Autodesk Inventor part; units mm, degrees
ref_plane "Plano de trabalho1" through (-163.24, 6, 12.15) normal (0, 0, 1) x (1, 0, 0)
ref_plane "Plano de trabalho2" through (-39.87, 6, 5) normal (0, 0, 1) x (1, 0, 0)
ref_plane "YZ Plane" through (0, 0, 0) normal (1, 0, 0) x (0, 1, 0)
sketch "Esboço1" plane through (0, 0, 0) normal (0, 1, 0) x (-1, 0, 0)
  line L0 (0, 5) -> (39.87, 5)
  line L1 (39.87, 5) -> (39.87, 12.15)
  line L2 (39.87, 12.15) -> (163.24, 12.15)
  line L3 (163.24, 12.15) -> (163.24, 7.27)
  line L4 (163.24, 7.27) -> (43.67, 7.27)
  line L5 (43.67, 7.27) -> (43.67, -0.21)
  line L6 (43.67, -0.21) -> (0, -0.21)
  line L7 (0, 5) -> (2.5, 5) construction
  line L8 (2.5, 5) -> (2.5, 1.56) construction
  line L9 (2.5, 1.56) -> (0, 1.56) construction
  line L10 (2.5, 1.56) -> (0, 5)
  line L11 (2.5, 1.56) -> (0, 1.56)
  line L12 (0, 1.56) -> (0, -0.21)
  point P0 (0, 0)
  dimension "d0" = 39.87
  dimension "d1" = 7.15
  dimension "d2" = 123.37
  dimension "d3" = 4.88
  dimension "d4" = 119.57
  dimension "d5" = 7.48
  dimension "d6" = 2.5
  dimension "d7" = 3.44
  dimension "d8" = 5.21
extrude "Extrusão1" add sketch "Esboço1" along normal mid plane 12
ref_plane "Plano de trabalho1" through (-163.24, 6, 12.15) normal (0, 0, 1) x (1, 0, 0)
ref_plane "Plano de trabalho2" through (-39.87, 6, 5) normal (0, 0, 1) x (1, 0, 0)
sketch "Esboço2" plane through (-163.24, 6, 12.15) normal (0, 0, 1) x (1, 0, 0)
  line L0 (123.37, 0) -> (123.37, -12) construction
  line L1 (123.37, -6) -> (110.26, -6) construction
  line L2 (0, 0) -> (0, -12) construction
  line L3 (0, -6) -> (3.56, -6) construction
  line L4 (110.26, -6) -> (0, -6) construction
  line L5 (3.56, -6) -> (110.26, -6) construction
  line L6 (6.785, -9.225) -> (107.035, -9.225)
  line L7 (107.035, -2.775) -> (6.785, -2.775)
  arc A0 (6.785, -2.775) -> (6.785, -9.225) centre (6.785, -6) ccw
  arc A1 (107.035, -9.225) -> (107.035, -2.775) centre (107.035, -6) ccw
  point P0 (163.24, -6)
  point P1 (55.13, -6)
  point P2 (56.91, -6)
  dimension "d13" = 13.11
  dimension "d14" = 3.56
  dimension "d16" = 6.45
extrude "Extrusão2" cut sketch "Esboço2" against normal blind 12
sketch "Esboço3" plane through (-39.87, 6, 5) normal (0, 0, 1) x (1, 0, 0)
  line L0 (-3.8, -12) -> (39.87, -12) construction
  line L1 (39.87, -12) -> (36.07, -12) construction
  line L2 (36.07, -12) -> (36.07, 0) construction
  line L3 (39.87, 0) -> (-3.8, 0) construction
  line L4 (39.87, -6) -> (39.87, -3.705) construction
  line L5 (39.87, 0) -> (39.87, -12) construction
  line L6 (39.87, -6) -> (39.87, -8.295) construction
  line L7 (39.87, -8.295) -> (36.07, -12)
  line L8 (39.87, -12) -> (36.07, -12)
  line L9 (39.87, -8.295) -> (39.87, -12)
  line L10 (36.07, 0) -> (39.87, -3.705)
  line L11 (39.87, 0) -> (39.87, -3.705)
  line L12 (39.87, 0) -> (36.07, 0)
  dimension "d19" = 3.8
  dimension "d20" = 2.295
  dimension "d21" = 2.295
extrude "Extrusão3" cut sketch "Esboço3" against normal blind 12
sketch "Esboço4" plane through (-39.87, 6, 5) normal (0, 0, 1) x (1, 0, 0)
  line L0 (39.87, -6) -> (34.49, -6) construction
  circle A0 centre (34.49, -6) radius 2.5
  dimension "d24" = 5.38
  dimension "d25" = 5
extrude "Extrusão4" add sketch "Esboço4" along normal blind 2
sketch "Esboço5" plane through (-5.38, 0, 7) normal (0, 0, 1) x (1, 0, 0)
  circle A0 centre (0, 0) radius 1
  point P0 (5.38, 0)
  dimension "d28" = 2
extrude "Extrusão5" add sketch "Esboço5" along normal blind 5.13
properties part number "pinças" material "Alumínio 6061"
Geometry check sheet. Reference: the model listing, model coordinates, mm. A direction names the side the tool comes from. Round coordinates to 2 decimals unless told otherwise and drop trailing zeros. Loops run counter-clockwise (first coordinate to the right, second up) from the corner with the lowest first, then second, coordinate; pieces in that order, holes last. Notation, with made-up numbers: (42.25, 28.5) - (71.25, 28.5) arc R11 ccw to (71.25, 32.5) - close; hole circle Ø9 at (-14.5, -1.75). An arc over 180 degrees is marked (long way). One line per question, with ' | ' between items. Start each with the question number.
1. Draft check along Y on faces 5 (the face through (-106, 3.225, 10)), 6 (the face through (-43.67, 0, 4)), 7 (the face through (-2.349, 4.585, 2.431)). Enter one of: released by +Y, released by -Y, zero draft, split by the parting line, or undercut.
2. Cross-section at D-D on z = 3.25. Record the cut outline in (x, y) (3 decimals), then the cut area to 3 significant figures.
3. Depth check by flat-ended pin: pin 1 (0.6 mm diameter, centred on x = -5, y = 0, fed in from +Z); pin 2 (2 mm diameter, centred on y = 2.5, z = 9, fed in from +X); pin 3 (2 mm diameter, centred on y = 2.5, z = 4.5, fed in from -X); pin 4 (5 mm diameter, centred on x = -100, y = 0, fed in from -Z) (1 decimal). Enter the tip coordinate at first touch or a pass-through.
4. Tool access check on faces 1 (the face through (-104, -4, 7.27)), 2 (the face through (-39.87, 0, 9)), 3 (the face through (-107, -3.225, 10)), 4 (the face through (-4, 0, 7)). Record the directions out of +Z, -Z, +X, -X, +Y, -Y that give a thin tool (end or side, any length) a straight path to the whole face; none if there is none.
5. Cross-section at B-B on x = -88. Record the cut outline in (y, z) (3 decimals).
6. Cross-section at C-C on x = -34.5. Record the cut outline in (y, z).
7. Cross-section at A-A on z = 10.25. Record the cut outline in (x, y) (3 decimals), then the cut area to 3 significant figures.
8. Scan lines: line 1 (Y direction, x = -87, z = 8.5) (3 decimals); line 2 (Z direction, x = -63.5, y = 4); line 3 (X direction, y = 3.75, z = 10). Record each from-to range of solid material in increasing order. Write a range as [from, to].
Taken from the geometry:
1) face 5: undercut | face 6: zero draft | face 7: released by +Y
2) outline: (-43.67, -6) - (-3.8, -6) - (-1.272, -3.535) - (-1.272, 3.535) - (-3.8, 6) - (-43.67, 6) - close | area: 503 mm²
3) pin 1: z = 12.13 | pin 2: x = -39.87 | pin 3: x = -43.67 | pin 4: through
4) face 1: -Z, -X, +Y, -Y | face 2: +Z, +Y, -Y | face 3: +Z, -Z | face 4: +Z
5) outline: (-6, 7.27) - (-3.225, 7.27) - (-3.225, 12.15) - (-6, 12.15) - close; (3.225, 7.27) - (6, 7.27) - (6, 12.15) - (3.225, 12.15) - close
6) outline: (-6, -0.21) - (6, -0.21) - (6, 5) - (-6, 5) - close
7) outline: (-163.24, -6) - (-39.87, -6) - (-39.87, 6) - (-163.24, 6) - close; circle Ø2 at (-5.38, 0); hole (-156.455, -3.225) - (-56.205, -3.225) arc R3.225 ccw to (-56.205, 3.225) - (-156.455, 3.225) arc R3.225 ccw to start | area: 804 mm²
8) line 1: [-6, -3.225], [3.225, 6] | line 2: [7.27, 12.15] | line 3: [-163.24, -39.87]
